Verification items for the finished model (mm, model axes). Face numbers are marked on the shaded views. A direction names the side the tool comes from. Give positions to 0.01 mm unless a question says otherwise; leave off trailing zeros. Write each loop counter-clockwise with the first axis right and the second up, starting at its lowest first coordinate (ties: lowest second). Pieces come first, ordered by that corner, then holes. Notation, with made-up numbers: (8.25, 70) - (52.25, 70) arc R14 cw to (52.25, 80) - close; hole circle Ø7 at (68.25, 1). An arc over 180 degrees is marked (long way). Put each result on its own line as item: value.
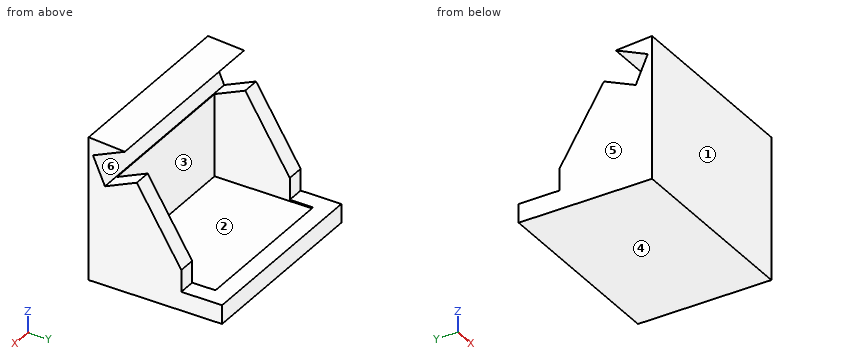
from build123d import *

# Parameters (mm, degrees)
F1_DEPTH = 22
F2_T     = 2
F3_DEPTH = 4
F4_DEPTH = 2.5


# Not quite as in the source:
# - a shell that OpenCascade refuses in one call is made with other operations: the cavity is built on its own and cut out
# - a feature names something its author has since deleted; it is built from what else it names


with BuildPart() as f1:
    # F0 (on Right) → F1 (new body)
    with BuildSketch(Plane.YZ):
        Polygon((-45.7758642733, 0), (-30.4509963948, 0), (-30.4525867105, 4.6551725827), (-35.1306907833, 4.6535744332), (-40.2460545301, 13.0035160109), (-41.6182950139, 16.1101743579), (-45.7758642733, 16.402374953), align=None)
    extrude(amount=F1_DEPTH)

    # F2: shell of thickness 2, made by hand


with BuildPart() as f2_core1:
    # F2_t2: copy of F1
    add(f1.part)

    # the walls: a layer under each face that stays
    f2_faces = [f2_core1.faces().sort_by_distance(p)[0] for p in [
        (11, -40.932174772, 14.5568451844),
        (11, -43.6970796436, 16.2562746555),
        (11, -45.7758642733, 8.2011874765),
        (11, -38.1134303341, 0),
        (11, -30.4517915527, 2.3275862914),
        (11, -32.7916387469, 4.6543735079),
        (0, -38.1134303341, 8.2011874765),
        (22, -38.1134303341, 8.2011874765),
    ]]
    thicken(f2_faces, amount=-F2_T, mode=Mode.SUBTRACT)


with BuildPart() as f1_1:
    add(f1.part)

    # what is left inside the walls is the cavity
    f2_cavity = [f2_core1.part.solids().sort_by_distance(p)[0] for p in [
        (14, -43.755864, 8.128439),
    ]]
    add(f2_cavity, mode=Mode.SUBTRACT)

    # F3 (cut): a face of the model
    f3_faces = [f1_1.faces().sort_by_distance(p)[0] for p in [
        (11, -40.932174772, 14.5568451844),
    ]]
    extrude(f3_faces, amount=-F3_DEPTH, mode=Mode.SUBTRACT)

    # F4 (cut): a face of the model
    f4_faces = [f1_1.faces().sort_by_distance(p)[0] for p in [
        (11, -32.7916387469, 4.6543735079),
    ]]
    extrude(f4_faces, amount=-F4_DEPTH, mode=Mode.SUBTRACT)


solid = f1_1.part
Q1. Release check for a two-part mould opening along Z. For the marked faces 3, 4, 5 and 6 record: released by +Z, released by -Z, zero draft, split by the parting line, or undercut.
Answers follow:
face 3: undercut
face 4: released by -Z
face 5: zero draft
face 6: undercut
Q2. Section check D-D, the plane z = 7.75. Record the cut outline in (x, y), plus the area to 3 significant figures.
Answers follow:
outline: (0, -45.78) - (22, -45.78) - (22, -37.03) - (20, -37.03) - (20, -43.78) - (2, -43.78) - (2, -37.03) - (0, -37.03) - close
area: 71.0 mm2
Q3. Go/stop test with flat-tipped pins: pin 1 Ø5.5 at (x, y) = (12, -36) entering from +Z; pin 2 Ø8 at (x, y) = (15.5, -44) entering from -Z; pin 3 Ø4.5 at (x, z) = (10, 6) entering from +Y; pin 4 Ø2 at (x, y) = (2.5, -36.5) entering from +Z. Record where each tip stops, or that it passes through.
Answers follow:
pin 1: stops at z = 2
pin 2: stops at z = 0
pin 3: stops at y = -43.78
pin 4: stops at z = 8.3
Q4. Scan lines: line 1 along X through (y, z) = (-41, 5); line 2 along Y through (x, z) = (21, 4.25); line 3 along Y through (x, z) = (3, 8.5). Record each from-to range of solid material in increasing order.
Answers follow:
line 1: x = 0 to 2, 20 to 22
line 2: y = -45.78 to -35.13
line 3: y = -45.78 to -43.78
Q5. Section check B-B, the plane z = 12.75. Record the cut outline in (x, y).
Answers follow:
outline: (0, -45.78) - (22, -45.78) - (22, -44.51) - (0, -44.51) - close; (0, -40.82) - (2, -40.82) - (2, -40.09) - (0, -40.09) - close; (20, -40.82) - (22, -40.82) - (22, -40.09) - (20, -40.09) - close
Q6. Section check A-A, the plane y = -44.5. Record the cut outline in (x, z).
Answers follow:
outline: (0, 0) - (22, 0) - (22, 12.73) - (0, 12.73) - close; (0, 14.84) - (22, 14.84) - (22, 16.31) - (0, 16.31) - close
Q7. Set-up check for the marked faces 1 and 2: record each of +Z, -Z, +X, -X, +Y, -Y from which the full face is reachable in a straight line by a thin tool's end or side.
Answers follow:
face 1: +Z, -Z, +X, -X, -Y
face 2: none
Q8. Section check C-C, the plane x = 20.5. Record the cut outline in (y, z) (3 decimals), plus the area to 3 significant figures.
Answers follow:
outline: (-45.776, 0) - (-30.451, 0) - (-30.452, 2.155) - (-35.13, 2.154) - (-35.131, 4.654) - (-40.246, 13.004) - (-43.905, 11.387) - (-45.277, 14.494) - (-41.618, 16.11) - (-45.776, 16.402) - close
area: 129 mm2
